```python
from build123d import *

# Parameters (mm, degrees)
SKETCH1_RX          = 50.023380752
SKETCH1_RY          = 25.011690376
BOSS_EXTRUDE1_DEPTH = 40
SKETCH2_W           = 53.048194423
SKETCH2_H           = 52.128277272
CUT_EXTRUDE1_DEPTH  = 40
SKETCH3_RX          = 45.004218106
SKETCH3_RY          = 20.025989305
CUT_EXTRUDE3_DEPTH  = 40
HANDLE_DEPTH        = 40
HANDLE_DEPTH_BACK   = 40
SKETCH4_W           = 7
SKETCH4_H           = 7
CUT_EXTRUDE4_START  = -27.500221438
CUT_EXTRUDE4_DEPTH  = 50.067195632
FILLET1_RADIUS      = 3.5
FILLET1_LENGTH      = 80
SKETCH6_W           = 3.5
SKETCH6_H           = 10
BOSS_EXTRUDE2_DEPTH = 25
SKETCH9_W           = 3.5
SKETCH9_H           = 10
BOSS_EXTRUDE3_DEPTH = 25


# Read off the part's stored shape, not the designer's step: Cut-Extrude4
with BuildPart() as part:
    # Sketch1 → Boss-Extrude1 (new body)
    with BuildSketch(Plane(origin=(0, 0, 0), x_dir=(1, 0, 0), z_dir=(0, 1, 0))):
        with Locations(Location((0, 0), (0, 0, -1.751851392))):
            Ellipse(SKETCH1_RX, SKETCH1_RY)
    extrude(amount=BOSS_EXTRUDE1_DEPTH)

    # Sketch2 → Cut-Extrude1 (cut)
    with BuildSketch(Plane(origin=(0, 40, 0), x_dir=(1, 0, 0), z_dir=(0, 1, 0))):
        with Locations((26.524365297, -1.043684065)):
            Rectangle(SKETCH2_W, SKETCH2_H)
    extrude(amount=-CUT_EXTRUDE1_DEPTH, mode=Mode.SUBTRACT)

    # Sketch3 → Cut-Extrude3 (cut)
    with BuildSketch(Plane(origin=(0, 40, 0), x_dir=(1, 0, 0), z_dir=(0, 1, 0))):
        with Locations(Location((0, 0), (0, 0, -0.784464251))):
            Ellipse(SKETCH3_RX, SKETCH3_RY)
    extrude(amount=-CUT_EXTRUDE3_DEPTH, mode=Mode.SUBTRACT)

    # Sketch4 → handle (add, two sides: drawn at the far end of the back side and taken through both)
    with BuildSketch(Plane(origin=(1.890919535, 40, 0), x_dir=(1, 0, 0), z_dir=(0, 1, 0)).offset(-HANDLE_DEPTH_BACK)):
        with Locations((-44.607863545, 1.046507327)):
            Rectangle(SKETCH4_W, SKETCH4_H)
    extrude(amount=HANDLE_DEPTH + HANDLE_DEPTH_BACK)

    # Cut-Extrude4 outline → Cut-Extrude4 (cut)
    with BuildSketch(Plane(origin=(1.890919535, 0, 2.453492673), x_dir=(1, 0, 0), z_dir=(0, 0, 1)).offset(CUT_EXTRUDE4_START)):
        with BuildLine():
            Line((-1.89065145, 40), (-41.022009989, 40))
            add(Edge.make_bspline(
                [(-41.022009989, 40), (-29.747385861, 24.075030507), (-18.472761733, 8.150061014), (-1.89065145, 8.183439673)],
                knots=[0, 0, 0, 0, 0.942635283, 0.942635283, 0.942635283, 0.942635283], degree=3))
            Line((-1.89065145, 8.183439673), (-1.89065145, 40))
        make_face()
    extrude(amount=CUT_EXTRUDE4_DEPTH, mode=Mode.SUBTRACT)

    # Fillet1: full round fillet: the end face becomes a half cylinder, R = half its width
    fillet1_face = Plane((-39.21694401, 40, -1.046507327), x_dir=(0, 1, 0), z_dir=(1, 0, 0))  # on the end face: x along it, z out of the body
    fillet1_slab = fillet1_face.offset(-FILLET1_RADIUS / 2) * Box(FILLET1_LENGTH, 2 * FILLET1_RADIUS, FILLET1_RADIUS, mode=Mode.PRIVATE)  # the body's end, R deep
    fillet1_round = Plane((-42.71694401, 40, -1.046507327), x_dir=(1, 0, 0), z_dir=(0, 1, 0)) * Cylinder(FILLET1_RADIUS, FILLET1_LENGTH, mode=Mode.PRIVATE)  # its axis R under the face
    add(fillet1_slab - fillet1_round, mode=Mode.SUBTRACT)

    # Sketch6 → Boss-Extrude2 (add)
    with BuildSketch(Plane.XY.offset(2.453492673)):
        with Locations((-44.46694401, 75)):
            Rectangle(SKETCH6_W, SKETCH6_H)
    extrude(amount=BOSS_EXTRUDE2_DEPTH)

    # Sketch9 → Boss-Extrude3 (add)
    with BuildSketch(Plane(origin=(0, 0, -4.546507327), x_dir=(-1, 0, 0), z_dir=(0, 0, -1))):
        with Locations((44.46694401, 75)):
            Rectangle(SKETCH9_W, SKETCH9_H)
    extrude(amount=BOSS_EXTRUDE3_DEPTH)


solid = part.part
```
The model under review builds one solid part; all positions refer to its coordinate system, in mm. A direction names the side the tool comes from. Give positions to 0.01 mm unless a question says otherwise; leave off trailing zeros. Loops run counter-clockwise (first coordinate to the right, second up) from the corner with the lowest first, then second, coordinate; pieces in that order, holes last. Notation, with made-up numbers: (25, 20.25) -> (33, 20.25) arc R29 cw to (33, 58.25) -> close; hole circle Ø5 at (79.25, 5). An arc over 180 degrees is marked (long way). Use CSV: the item, a comma, the result in double quotes.
1. Consider section A-A, the plane y = 66. Write out the cut boundary in (x, z), then the cut area to 3 significant figures.
Result:
outline,"(-46.22, -4.55) -> (-42.72, -4.55) arc R3.5 ccw to (-42.72, 2.45) -> (-46.22, 2.45) -> close"
area,"43.7 mm²"
2. The part is to be moulded in two halves that separate along Z. For faces 6 (the face through (-44, 42, -4.547)), 7 (the face through (-44, 75, -29.547)), 8 (the face through (-47, 40, -1)), say which applies: +Z half, -Z half, draft (parallel to the pull), parting line (faces both ways), or undercut.
Result:
face 6,"undercut"
face 7,"-Z half"
face 8,"draft"
3. For P1, Ø5, axis at y = 26, z = -10, coming from the +X side; P2, Ø11, axis at y = 76.5, z = -20, coming from the +X side; P3, Ø4, axis at x = -44, y = 31, coming from the +Z side, all flat-tipped, find the tip position at first contact; note any pin that passes through.
Result:
P1,"stops at x = -35.85"
P2,"stops at x = -42.72"
P3,"stops at z = 12.62"
4. To check wall thickness, follow probe 1 along X at (y, z) = (72, -23); probe 2 along Z at (x, y) = (-41.5, 25.5); probe 3 along X at (y, z) = (6, 7). State the ranges of each line that lie inside material, in increasing order. Write a range as from..to.
Result:
probe 1,"x = -46.22..-42.72"
probe 2,"z = -14.91..-8.2, -4.33..2.24, 7.29..13.01"
probe 3,"x = -47.32..-41.76"
5. Machinability: for faces 1 (the face through (-44, 70, -17)), 2 (the face through (-42.717, 75, 15)), 3 (the face through (-44, 70, 15)), 4 (the face through (-42.717, 75, -17)), 5 (the face through (-46.217, 69, -1)), which of the approach directions +Z, -Z, +X, -X, +Y, -Y give a long, thin tool a straight path to every point of the face, cutting with its end or side? Answer none if there is none.
Result:
face 1,"-Z, +X, -X"
face 2,"+Z, +X, +Y"
face 3,"+Z, +X, -X"
face 4,"-Z, +X, +Y"
face 5,"+Z, -Z, -X, +Y"
